Could you check a few things on this model? Use its own coordinates, in mm. A direction names the side the tool comes from. Round coordinates to 2 decimals unless told otherwise and drop trailing zeros. Write each loop counter-clockwise with the first axis right and the second up, starting at its lowest first coordinate (ties: lowest second). Pieces come first, ordered by that corner, then holes. Notation, with made-up numbers: (88, 58) - (92, 58) arc R29 cw to (92, 83) - close; hole circle Ø9 at (28.5, 62.25). An arc over 180 degrees is marked (long way). Write each question's results on one line, items separated by ' | '. Start each with the question number.
(1) Imagine slicing it at B-B on z = 4.25. Write out the boundary of the cut face in (x, y).
(2) Imagine slicing it at C-C on y = 3.5. Write out the boundary of the cut face in (x, z).
(3) Thinking about a two-plate mould opening in X: for faces 6 (the flat face through (5, 8.104, 1)), 7 (the cylindrical face through (-11.325, 4.726, 1.454)), 8 (the cylindrical face through (-12.906, 6.115, 1.479)), which applies, +X half, -X half, draft (parallel to the pull), parting line (faces both ways), or undercut?
(4) Imagine slicing it at D-D on x = 7.5. Write out the boundary of the cut face in (y, z), then the cut area to 3 significant figures.
(5) For P1, Ø1.5, axis at y = 8, z = 4, coming from the -X side; P2, Ø2, axis at x = -5.5, z = 2.5, coming from the +Y side; P3, Ø3, axis at x = -2.5, y = 5.5, coming from the -Z side, each with a flat end and sliding along its axis, tell me the tip position at first contact or that it passes through.
(6) Please list where these lines run through material, in increasing order: line 1 (X direction, y = 4.25, z = 4.5); line 2 (X direction, y = 6.25, z = -1.5); line 3 (Y direction, x = -5, z = 1). Write a range as [from, to].
(7) On a 3-axis mill with a long thin cutter (end or side, diameter ignored), from which of +Z, -Z, +X, -X, +Y, -Y can I reach the whole of each face in a straight line? I mean faces 1 (the flat face through (-8, 8, 4.75)), 2 (the flat face through (10.922, 6, 5)), 3 (the cylindrical face through (-11.96, 4.24, 3.86)), 4 (the flat face through (10.922, 6, -2)), 5 (the flat face through (-8, 4, -1.75)). Say none if no direction works.
(8) Imagine slicing it at A-A on y = 5.25. Write out the boundary of the cut face in (x, z), then the cut area to 3 significant figures.
```python
from build123d import *

# Parameters (mm, degrees)
F0_R      = 2.1
F1_DEPTH  = 3
F2_W      = 7.8759681508
F2_H      = 2.3975596942
F2_H_2    = 2.4024403058
F3_DEPTH  = 25
F2_H_3    = 4.2
F4_DEPTH  = 5
F5_DEPTH  = 8
F7_DEPTH  = 25
F8_R      = 2.9
F8_R_2    = 2.1
F9_DEPTH  = 1.75
F10_R     = 2.9
F10_R_2   = 2.1
F11_DEPTH = 1.75


with BuildPart() as f1:
    # F0 (on Top) → F1 (new body)
    with BuildSketch(Plane.XY):
        Polygon((18.7982146922, 10.5015123645), (10.9222465414, 10.5015123645), (10.9222465414, 8.1039526702), (10.9222465414, 3.9039526702), (10.9222465414, 1.5015123645), (18.7982146922, 1.5015123645), align=None)
        with BuildLine():
            Line((10.9222465414, 3.9039526702), (10.9222465414, 8.1039526702))
            Line((10.9222465414, 8.1039526702), (-7.1777534586, 8.1039526702))
            ThreePointArc((-7.1777534586, 8.1039526702), (-12.9081768095, 6.0039526702), (-7.1777534586, 3.9039526702))
            Line((-7.1777534586, 3.9039526702), (10.9222465414, 3.9039526702))
        make_face()
        with Locations((-9.6581768095, 6.0039526702)):
            Circle(F0_R, mode=Mode.SUBTRACT)
    extrude(amount=F1_DEPTH)

    # F2 (on face) → F3 (cut)
    with BuildSketch(Plane.XY.offset(3)):
        with Locations((14.8602306168, 9.3027325174)):
            Rectangle(F2_W, F2_H)
        with Locations((14.8602306168, 2.7027325174)):
            Rectangle(F2_W, F2_H_2)
    extrude(amount=-F3_DEPTH, mode=Mode.SUBTRACT)

    # F2 (on face) → F4 (join)
    with BuildSketch(Plane.XY.offset(3)):
        with Locations((14.8602306168, 6.0039526702)):
            Rectangle(F2_W, F2_H_3)
    extrude(amount=F4_DEPTH)

    # F2 (on face) → F5 (join)
    with BuildSketch(Plane.XY.offset(3)):
        with Locations((14.8602306168, 6.0039526702)):
            Rectangle(F2_W, F2_H_3)
    extrude(amount=-F5_DEPTH)

    # F6 (on face) → F7 (cut)
    with BuildSketch(Plane(origin=(0, 8.1039526702, 0), x_dir=(-1, 0, 0), z_dir=(0, 1, 0))):
        with BuildLine():
            ThreePointArc((-10.9222465414, -4.0903488442), (-13.1232466414, 1.5), (-10.9222465414, 7.0903488442))
            Line((-10.9222465414, 7.0903488442), (-10.9222465414, 8))
            Line((-10.9222465414, 8), (-18.7982146922, 8))
            Line((-18.7982146922, 8), (-18.7982146922, -5))
            Line((-18.7982146922, -5), (-10.9222465414, -5))
            Line((-10.9222465414, -5), (-10.9222465414, -4.0903488442))
        make_face()
    extrude(amount=-F7_DEPTH, mode=Mode.SUBTRACT)

    # F8 (on face) → F9 (join)
    with BuildSketch(Plane(origin=(0, 0, 0), x_dir=(1, 0, 0), z_dir=(0, 0, -1))):
        with Locations((-9.6581768095, -6.0039526702)):
            Circle(F8_R)
        with Locations((-9.6581768095, -6.0039526702)):
            Circle(F8_R_2, mode=Mode.SUBTRACT)
    extrude(amount=F9_DEPTH)

    # F10 (on face) → F11 (join)
    with BuildSketch(Plane.XY.offset(3)):
        with Locations((-9.6581768095, 6.0039526702)):
            Circle(F10_R)
        with Locations((-9.6581768095, 6.0039526702)):
            Circle(F10_R_2, mode=Mode.SUBTRACT)
    extrude(amount=F11_DEPTH)


solid = f1.part
```
Response:
1) outline: circle Ø5.8 at (-9.66, 6); (10.92, 3.9) - (12.65, 3.9) - (12.65, 8.1) - (10.92, 8.1) - close; hole circle Ø4.2 at (-9.66, 6)
2) outline: (-11.73, 0) - (-11.12, 0) - (-11.12, -1.75) - (-8.2, -1.75) - (-8.2, 0) - (-7.59, 0) - (-7.59, 3) - (-8.2, 3) - (-8.2, 4.75) - (-11.12, 4.75) - (-11.12, 3) - (-11.73, 3) - close
3) face 6: draft | face 7: undercut | face 8: parting line
4) outline: (3.9, 0) - (8.1, 0) - (8.1, 3) - (3.9, 3) - close | area: 12.6 mm²
5) P1: x = -12.28 | P2: y = 8.1 | P3: z = 0
6) line 1: [-11.97, -10.81], [-8.5, -7.35], [10.92, 12.55] | line 2: [-12.55, -11.74], [-7.57, -6.77], [10.92, 12.55] | line 3: [3.9, 8.1]
7) face 1: +Z, -X, +Y, -Y | face 2: +Z, +Y, -Y | face 3: +Z | face 4: -Z, +Y, -Y | face 5: -Z, -X, +Y, -Y
8) outline: (-12.82, 0) - (-12.46, 0) - (-12.46, -1.75) - (-11.62, -1.75) - (-11.62, 4.75) - (-12.46, 4.75) - (-12.46, 3) - (-12.82, 3) - close; (-7.7, -1.75) - (-6.86, -1.75) - (-6.86, 0) - (10.92, 0) - (10.92, -4.09) arc R8.2 ccw to (10.92, 7.09) - (10.92, 3) - (-6.86, 3) - (-6.86, 4.75) - (-7.7, 4.75) - close | area: 82.3 mm²
